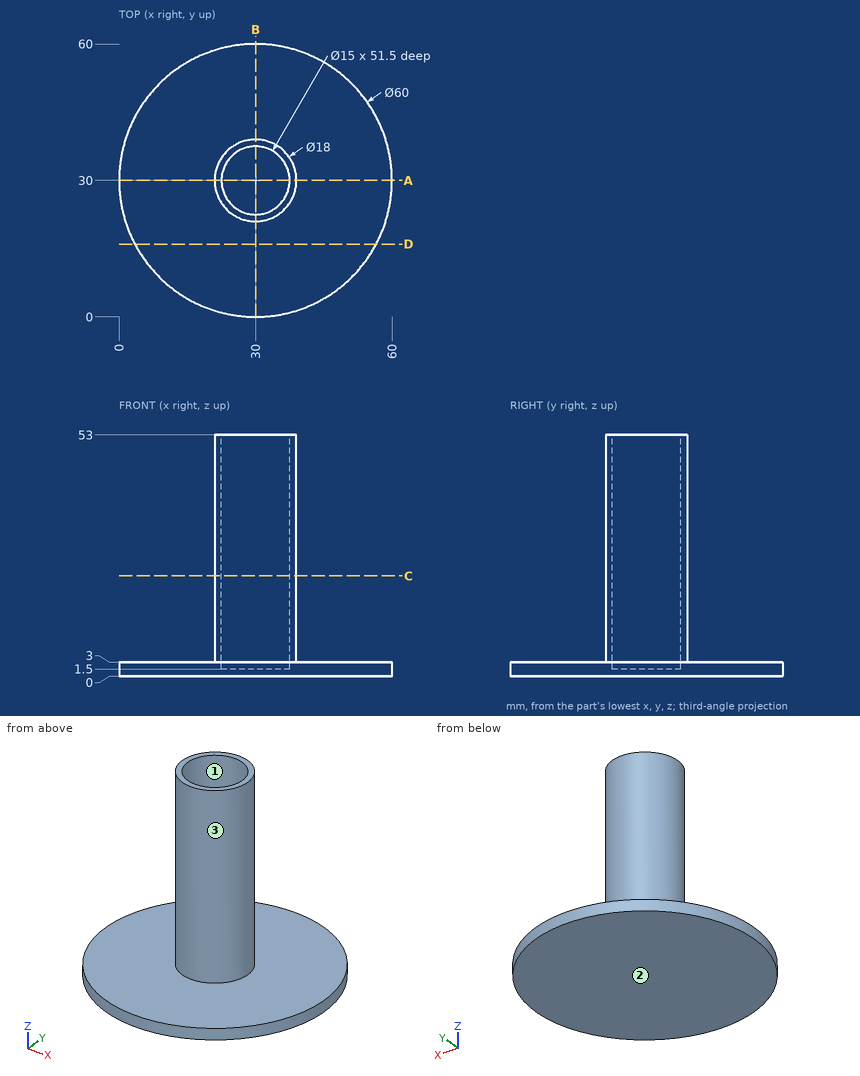
Input: dimensioned drawing with shaded views. Units: mm. Origin: part minimum x, y, z. Round coordinates to 2 decimals unless told otherwise and drop trailing zeros. Loops run counter-clockwise (first coordinate to the right, second up) from the corner with the lowest first, then second, coordinate; pieces in that order, holes last.
1) Material intervals for line 1 (Y direction, x = 30, z = 26); line 2 (Z direction, x = 22.5, y = 23); line 3 (X direction, y = 26, z = 25.5), sorted ascending.
Ans:
line 1: y = 21 to 22.5, 37.5 to 39
line 2: z = 0 to 3
line 3: x = 21.94 to 23.66, 36.34 to 38.06
2) Section query D-D on y = 16. Return the cut outline in (x, z).
Ans:
outline: (3.47, 0) - (56.53, 0) - (56.53, 3) - (3.47, 3) - close
3) Pull-direction query (Y, two-part tool) for the marked faces 1, 2 and 3; classes: released by +Y, released by -Y, zero draft, split by the parting line, or undercut.
Ans:
face 1: undercut
face 2: zero draft
face 3: split by the parting line
4) Section query C-C on z = 22. Return the cut outline in (x, y).
Ans:
outline: circle Ø18 at (30, 30); hole circle Ø15 at (30, 30)
5) Section query A-A on y = 30. Return the cut outline in (x, z), plus the area to 4 significant figures.
Ans:
outline: (0, 0) - (60, 0) - (60, 3) - (39, 3) - (39, 53) - (37.5, 53) - (37.5, 1.5) - (22.5, 1.5) - (22.5, 53) - (21, 53) - (21, 3) - (0, 3) - close
area: 307.5 mm2
6) Pin query (flat end, axial travel): pin 1 (2 mm diameter, centred on y = 33.5, z = 30.5, fed in from -X); pin 2 (12 mm diameter, centred on y = 34, z = 12.5, fed in from +X); pin 3 (4.5 mm diameter, centred on x = 28, y = 28.5, fed in from +Z). Return the tip coordinate at first contact, or that it passes through.
Ans:
pin 1: stops at x = 21.35
pin 2: stops at x = 39
pin 3: stops at z = 1.5
